Geometry check sheet. Reference: drawing and pictorial views, mm from the part's lowest x, y, z. Give positions to 0.01 mm unless a question says otherwise; leave off trailing zeros. Loops run counter-clockwise (first coordinate to the right, second up) from the corner with the lowest first, then second, coordinate; pieces in that order, holes last. Notation, with made-up numbers: (-16, -21) - (39, -21) arc R25 ccw to (39, 15) - close; hole circle Ø2 at (7.5, -22.75). An arc over 180 degrees is marked (long way). Answer in a Markdown table with one row per item. Add a question column.
(1) Draft check along Y on the marked faces 1, 2, 3 and 4. Enter one of: released by +Y, released by -Y, zero draft, split by the parting line, or undercut.
(2) Thickness scan on L1, parallel to X at y = 41.5, z = 2.85; L2, parallel to Y at x = 15, z = 1.8. Record the ranges inside material, lowest first.
(3) Go/stop test with a flat-tipped pin: P1, Ø6, axis at x = 15.5, y = 44.5, coming from the +Z side. Record where the tip stops, or that it passes through.
(4) Sectioned sample at B-B on x = 15. Enter the section's corners in (y, z).
(5) Sectioned sample at C-C on z = 2.15. Enter the section's corners in (x, y), then the cut area to 3 significant figures.
(6) Sectioned sample at A-A on y = 19. Enter the section's corners in (x, z), then the cut area to 3 significant figures.
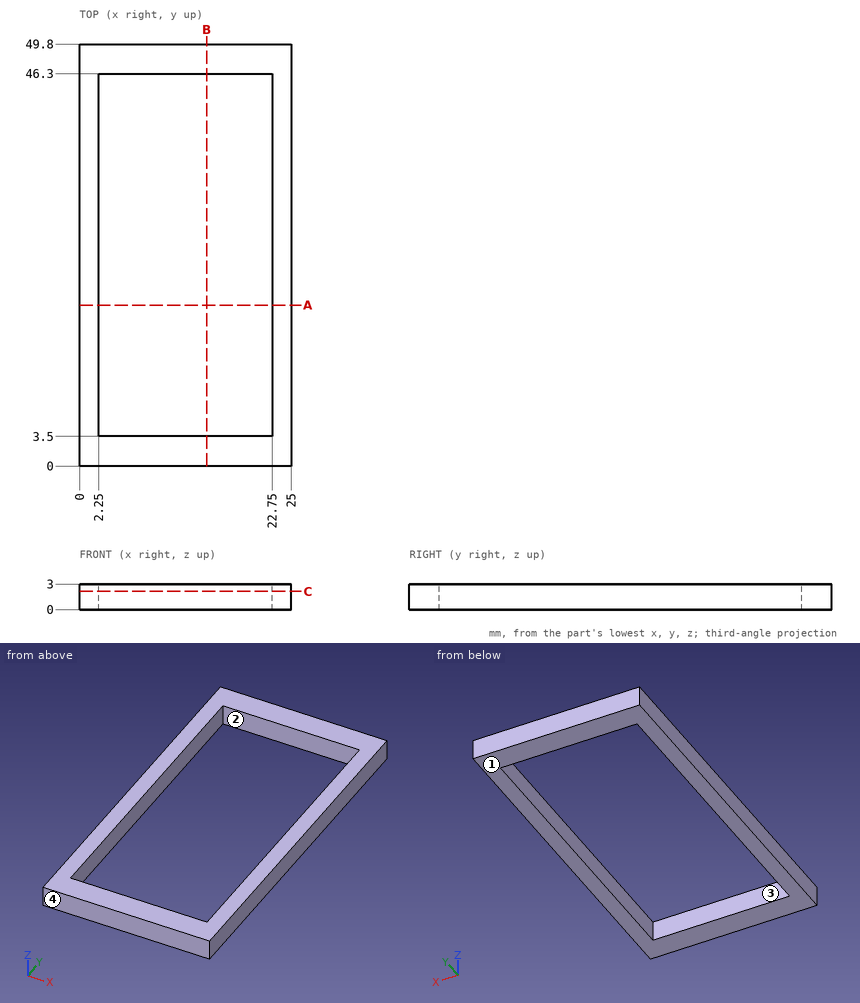
Reply:
| question | item | result |
|---|---|---|
| 1 | face 1 | zero draft |
| 1 | face 2 | undercut |
| 1 | face 3 | undercut |
| 1 | face 4 | released by -Y |
| 2 | L1 | 0 to 2.25, 22.75 to 25 |
| 2 | L2 | 0 to 3.5, 46.3 to 49.8 |
| 3 | P1 | z = 3 |
| 4 | outline | (0, 0) - (3.5, 0) - (3.5, 3) - (0, 3) - close; (46.3, 0) - (49.8, 0) - (49.8, 3) - (46.3, 3) - close |
| 5 | outline | (0, 0) - (25, 0) - (25, 49.8) - (0, 49.8) - close; hole (2.25, 3.5) - (22.75, 3.5) - (22.75, 46.3) - (2.25, 46.3) - close |
| 5 | area | 368 mm^2 |
| 6 | outline | (0, 0) - (2.25, 0) - (2.25, 3) - (0, 3) - close; (22.75, 0) - (25, 0) - (25, 3) - (22.75, 3) - close |
| 6 | area | 13.5 mm^2 |
